The model under review builds one solid part; all positions refer to its coordinate system, in mm. Face numbers are marked on the shaded views. A direction names the side the tool comes from. Round coordinates to 2 decimals unless told otherwise and drop trailing zeros. Order: outer loops, then holes, each group sorted by start corner. A loop starts at its lowest first (then second) coordinate and runs counter-clockwise, first axis right, second up. Notation, with made-up numbers: M 37.25,-11.5 L 78.25,-11.5 A15 cw 78.25,2.5 Z; hole C 24.25,-34.5 d9. An arc over 180 degrees is marked long. One line per item, written item: value. Start each with the question number.
from build123d import *

# Parameters (mm, degrees)
ESQUISSE1_R             = 5
BOSS_EXTRU_1_DEPTH      = 20
ENL_V_MAT_EXTRU_1_REACH = 51.891
ESQUISSE2_R             = 3.3
ESQUISSE3_R             = 5.4
ENL_V_MAT_EXTRU_2_DEPTH = 5
ESQUISSE4_R             = 13
ENL_V_MAT_EXTRU_3_DEPTH = 6
ENL_V_START             = -6
ESQUISSE5_R             = 13
ENL_V_MAT_EXTRU_4_DEPTH = 6


with BuildPart() as part:
    # Esquisse1 → Boss.-Extru.1 (new body)
    with BuildSketch(Plane.XY):
        Polygon((-27.861974124, -13.935926773), (32.138025876, -13.935926773), (32.138025876, 18.564073227), (19.138025876, 18.564073227), (19.138025876, 29.064073227), (-14.861974124, 29.064073227), (-14.861974124, 18.564073227), (-27.861974124, 18.564073227), align=None)
        with Locations((2.138025876, 11.064073227)):
            Circle(ESQUISSE1_R, mode=Mode.SUBTRACT)
    extrude(amount=BOSS_EXTRU_1_DEPTH)

    # Esquisse2 → Enlèv. mat.-Extru.1 (cut, up to next)
    with BuildSketch(Plane(origin=(0, 18.564073227, 0), x_dir=(1, 0, 0), z_dir=(0, 1, 0)), mode=Mode.PRIVATE) as enl_v_mat_extru_1_sk1:
        with Locations(Location((25.138025876, -10, 0), (0, 0, 270))):
            Circle(ESQUISSE2_R)
    enl_v_mat_extru_1_tool1 = extrude(enl_v_mat_extru_1_sk1.sketch, amount=-ENL_V_MAT_EXTRU_1_REACH, mode=Mode.PRIVATE) & part.part
    # Esquisse2 → Enlèv. mat.-Extru.1 (cut, up to next)
    with BuildSketch(Plane(origin=(0, 18.564073227, 0), x_dir=(1, 0, 0), z_dir=(0, 1, 0)), mode=Mode.PRIVATE) as enl_v_mat_extru_1_sk2:
        with Locations(Location((-20.861974124, -10, 0), (0, 0, 270))):
            Circle(ESQUISSE2_R)
    enl_v_mat_extru_1_tool2 = extrude(enl_v_mat_extru_1_sk2.sketch, amount=-ENL_V_MAT_EXTRU_1_REACH, mode=Mode.PRIVATE) & part.part
    add(enl_v_mat_extru_1_tool1.solids().sort_by_distance((25.138026, 18.564073, 10))[0], mode=Mode.SUBTRACT)
    add(enl_v_mat_extru_1_tool2.solids().sort_by_distance((-20.861974, 18.564073, 10))[0], mode=Mode.SUBTRACT)

    # Esquisse3 → Enlèv. mat.-Extru.2 (cut)
    with BuildSketch(Plane(origin=(0, 18.564073227, 0), x_dir=(1, 0, 0), z_dir=(0, 1, 0))):
        with Locations(Location((25.138025876, -10, 0), (0, 0, 270))):
            Circle(ESQUISSE3_R)
        with Locations(Location((-20.861974124, -10, 0), (0, 0, 270))):
            Circle(ESQUISSE3_R)
    extrude(amount=-ENL_V_MAT_EXTRU_2_DEPTH, mode=Mode.SUBTRACT)

    # Esquisse4 → Enlèv. mat.-Extru.3 (cut)
    with BuildSketch(Plane.XY.offset(20)):
        with Locations((2.138025876, 11.064073227)):
            Circle(ESQUISSE4_R)
    extrude(amount=-ENL_V_MAT_EXTRU_3_DEPTH, mode=Mode.SUBTRACT)

    # Esquisse5 → Enlèv. mat.-Extru.4 (cut)
    with BuildSketch(Plane(origin=(0, 0, 0), x_dir=(-1, 0, 0), z_dir=(0, 0, -1)).offset(ENL_V_START)):
        with Locations(Location((-2.138025876, 11.064073227, 0), (0, 0, 180))):
            Circle(ESQUISSE5_R)
    extrude(amount=ENL_V_MAT_EXTRU_4_DEPTH, mode=Mode.SUBTRACT)


solid = part.part
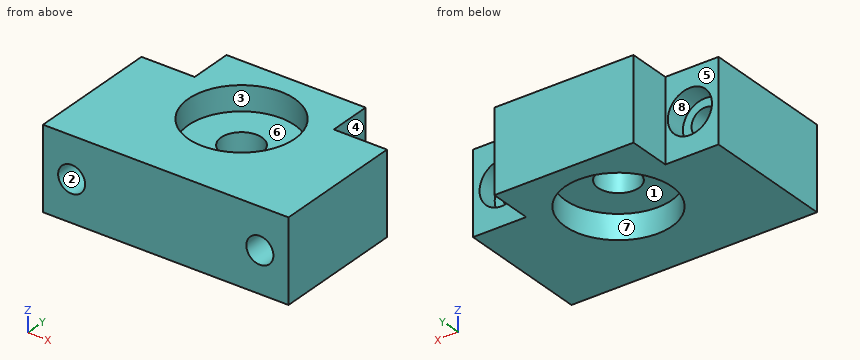
Item 1: Consider section C-C, the plane x = 9. Give the boundary of the cut face in (y, z), then the cut area to 3 significant figures.
Item 2: Consider section D-D, the plane z = 2.25. Give the boundary of the cut face in (x, y), then the cut area to 3 significant figures.
Item 3: Consider section B-B, the plane y = 2.5. Give the boundary of the cut face in (x, z), then the cut area to 3 significant figures.
Item 4: The part is to be moulded in two halves that separate along Z. For the marked faces 1, 2 and 3, say which applies: pulls with the +Z half, pulls with the -Z half, needs draft (parallel to the pull), parting line crosses it, or undercut.
Item 5: Consider section A-A, the plane z = 11.5. Give the boundary of the cut face in (x, y).
Item 6: Clearance check with flat-ended pins moving along their axes: P1, Ø11.5, axis at x = 2.14, y = 11.06, coming from the +Z side; P2, Ø3, axis at y = 23.5, z = 9.5, coming from the +X side; P3, Ø6.5, axis at x = -20.86, z = 10, coming from the +Y side; P4, Ø7.5, axis at x = -20.86, z = 10, coming from the +Y side. State where each tip first meets the part, or that it passes through.
Item 7: Machinability: for the marked faces 4, 5, 6, 7 and 8, which of the approach directions +Z, -Z, +X, -X, +Y, -Y give a long, thin tool a straight path to every point of the face, cutting with its end or side? Answer none if there is none.
Item 8: Wall thickness on L1, parallel to Y at x = 2, z = 2.75; L2, parallel to X at y = -7.75, z = 10; L3, parallel to Z at x = 25, y = 8.5: over which ranges is each line inside the solid? List them lowest first.
Computed:
1. outline: M -13.94,0 L 0.02,0 L 0.02,6 L 22.11,6 L 22.11,0 L 29.06,0 L 29.06,20 L 22.11,20 L 22.11,14 L 0.02,14 L 0.02,20 L -13.94,20 Z
1. area: 595 mm^2
2. outline: M -27.86,-13.94 L 32.14,-13.94 L 32.14,18.56 L 19.14,18.56 L 19.14,29.06 L -14.86,29.06 L -14.86,18.56 L -27.86,18.56 Z; hole C 2.14,11.06 d26
2. area: 1,780 mm^2
3. outline: M -27.86,0 L -7.64,0 L -7.64,6 L 11.92,6 L 11.92,0 L 32.14,0 L 32.14,20 L 11.92,20 L 11.92,14 L -7.64,14 L -7.64,20 L -27.86,20 Z; hole C -20.86,10 d6.6; hole C 25.14,10 d6.6
3. area: 897 mm^2
4. face 1: pulls with the -Z half
4. face 2: undercut
4. face 3: needs draft
5. outline: M -27.86,-13.94 L -23.8,-13.94 L -23.8,13.56 L -26.05,13.56 L -26.05,18.56 L -27.86,18.56 Z; M -17.92,-13.94 L 22.2,-13.94 L 22.2,13.56 L 19.95,13.56 L 19.95,18.56 L 19.14,18.56 L 19.14,29.06 L -14.86,29.06 L -14.86,18.56 L -15.67,18.56 L -15.67,13.56 L -17.92,13.56 Z; M 28.08,-13.94 L 32.14,-13.94 L 32.14,18.56 L 30.33,18.56 L 30.33,13.56 L 28.08,13.56 Z; hole C 2.14,11.06 d10
6. P1: stops at z = 14
6. P2: stops at x = 19.14
6. P3: passes through
6. P4: stops at y = 13.56
7. face 4: +Z, -Z, +X, +Y
7. face 5: +Z, -Z, -X, +Y
7. face 6: +Z
7. face 7: -Z
7. face 8: +Y
8. L1: y = -13.94 to -1.94, 24.06 to 29.06
8. L2: x = -27.86 to -24.16, -17.56 to 21.84, 28.44 to 32.14
8. L3: z = 0 to 6.7, 13.3 to 20
